For this review, use the dimensioned drawing (mm, ordinates from the lowest corner) and the shaded views. A direction names the side the tool comes from. Round coordinates to 2 decimals unless told otherwise and drop trailing zeros. Write each loop counter-clockwise with the first axis right and the second up, starting at its lowest first coordinate (ties: lowest second). Pieces come first, ordered by that corner, then holes. Notation, with made-up numbers: M 43,9.5 L 83,9.5 A20 cw 83,18.5 Z; hole C 26.5,19.5 d11. An arc over 180 degrees is marked long. One line per question, with ' | ' between items. Start each with the question number.
Item 1: Add section D-D, the plane x = 20. State the section outline as (y, z) points.
Item 2: Add section B-B, the plane y = 10.5. State the section outline as (x, z) points, and give its area (3 significant figures).
Item 3: For L1, parallel to X at y = 2.85, z = 10; L2, parallel to Z at x = 30, y = 1.95; L3, parallel to Z at x = 30, y = 0.45, list the stretches that pass through material, from the lowest coordinate up.
Item 4: Draft analysis for pull direction Z (two halves, no side actions). For the marked faces 1, 2, 3 and 4, state which applies: released by +Z, released by -Z, zero draft, split by the parting line, or undercut.
Item 5: Add section A-A, the plane x = 30. State the section outline as (y, z) points.
Item 6: Machinability: for the marked faces 5, 6 and 7, which of the approach directions +Z, -Z, +X, -X, +Y, -Y give a long, thin tool a straight path to every point of the face, cutting with its end or side? Answer none if there is none.
Item 7: Insertion check: pin 1 Ø1.5 at (y, z) = (11.5, 13) entering from +X; pin 2 Ø8 at (x, z) = (10, 10) entering from +Y; pin 3 Ø2 at (y, z) = (10.5, 8) entering from -X. Each pin has a flat end and moves straight along its axis. Give the tip position at first contact, or say it passes through.
Item 8: Add section C-C, the plane z = 11.5. State the section outline as (x, y) points, and give its area (3 significant figures).
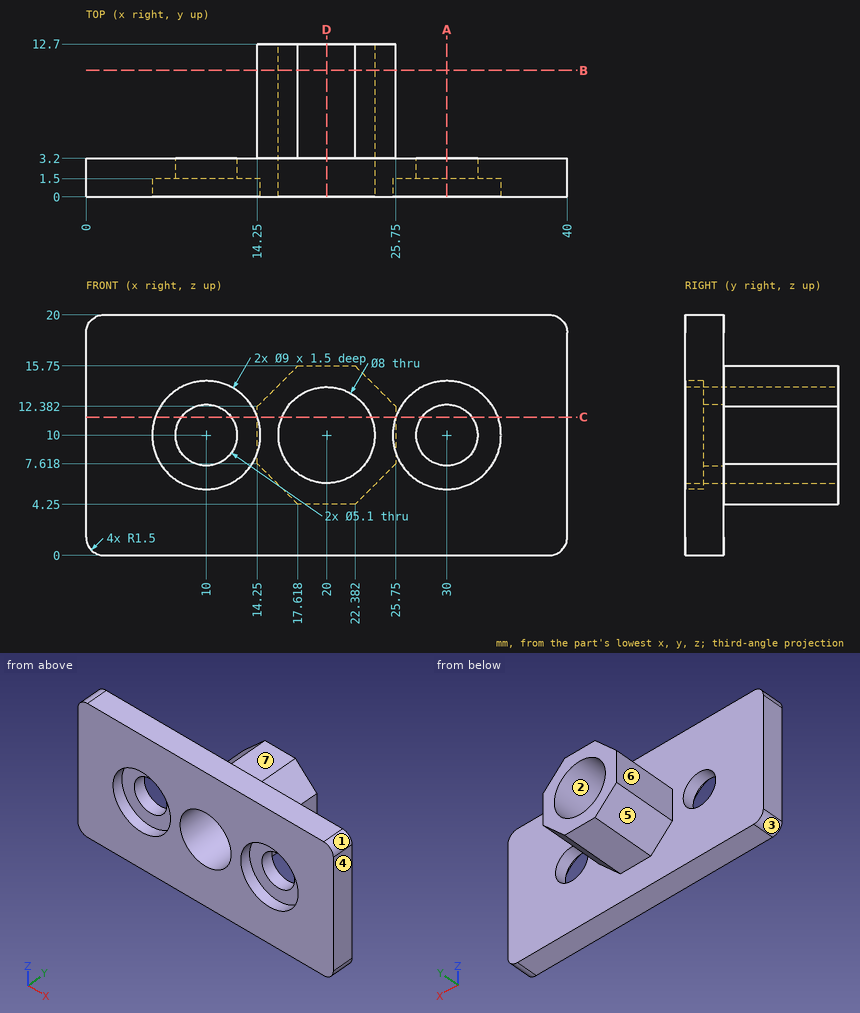
Computed values:
1) outline: M 0,0 L 3.2,0 L 3.2,4.25 L 12.7,4.25 L 12.7,6 L 0,6 Z; M 0,14 L 12.7,14 L 12.7,15.75 L 3.2,15.75 L 3.2,20 L 0,20 Z
2) outline: M 14.25,7.62 L 17.62,4.25 L 22.38,4.25 L 25.75,7.62 L 25.75,12.38 L 22.38,15.75 L 17.62,15.75 L 14.25,12.38 Z; hole C 20,10 d8 | area: 59.3 mm^2
3) L1: x = 0 to 7.45, 12.55 to 16, 24 to 27.45, 32.55 to 40 | L2: z = 0 to 7.45, 12.55 to 20 | L3: z = 0 to 5.5, 14.5 to 20
4) face 1: released by +Z | face 2: undercut | face 3: released by -Z | face 4: zero draft
5) outline: M 0,0 L 3.2,0 L 3.2,7.45 L 1.5,7.45 L 1.5,5.5 L 0,5.5 Z; M 0,14.5 L 1.5,14.5 L 1.5,12.55 L 3.2,12.55 L 3.2,20 L 0,20 Z
6) face 5: -Z, -X, +Y | face 6: +Z, -Z, -X, +Y | face 7: +Z, +X, -X, +Y
7) pin 1: stops at x = 25.75 | pin 2: stops at y = 3.2 | pin 3: stops at x = 14.25
8) outline: M 0,0 L 5.76,0 L 5.76,1.5 L 7.94,1.5 L 7.94,3.2 L 0,3.2 Z; M 12.06,1.5 L 14.24,1.5 L 14.24,0 L 16.29,0 L 16.29,12.7 L 14.25,12.7 L 14.25,3.2 L 12.06,3.2 Z; M 23.71,0 L 25.76,0 L 25.76,1.5 L 27.94,1.5 L 27.94,3.2 L 25.75,3.2 L 25.75,12.7 L 23.71,12.7 Z; M 32.06,1.5 L 34.24,1.5 L 34.24,0 L 40,0 L 40,3.2 L 32.06,3.2 Z | area: 104 mm^2
